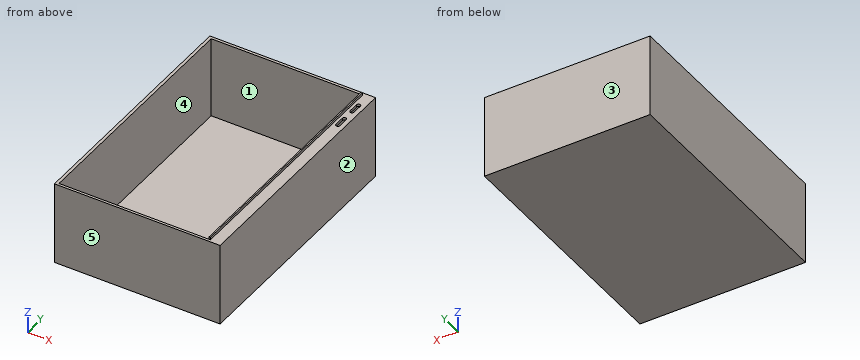
```python
from build123d import *

# Parameters (mm, degrees)
F0_W     = 406.4
F0_H     = 609.6
F1_DEPTH = 203.2
F2_W     = 368.3
F2_H     = 596.9
F3_DEPTH = 199.39
F5_DEPTH = 25.4
F7_DEPTH = 25.4
F8_W     = 3.175
F8_H     = 596.9
F9_DEPTH = 6.35


with BuildPart() as f1:
    # F0 (on Top) → F1 (new body)
    with BuildSketch(Plane.XY):
        Rectangle(F0_W, F0_H)
    extrude(amount=F1_DEPTH)

    # F2 (on face) → F3 (cut)
    with BuildSketch(Plane.XY.offset(203.2)):
        with Locations((-11.712919, -0.323749)):
            Rectangle(F2_W, F2_H)
    extrude(amount=-F3_DEPTH, mode=Mode.SUBTRACT)

    # F4 (on face) → F5 (cut)
    with BuildSketch(Plane(origin=(172.437081, 0, 0), x_dir=(0, -1, 0), z_dir=(-1, 0, 0))):
        Polygon((-298.126251, 196.85), (-298.126251, 3.81), (298.773749, 3.81), (298.773749, 196.85), (-77.169992, 196.85), align=None)
    extrude(amount=-F5_DEPTH, mode=Mode.SUBTRACT)

    # F6 (on face) → F7 (cut)
    with BuildSketch(Plane.XY.offset(203.2)):
        with BuildLine():
            Line((192.28287, 237.560081), (192.282062, 262.872214))
            ThreePointArc((192.282062, 262.872214), (187.564229, 267.722228), (182.75787, 262.959929))
            Line((182.75787, 262.959929), (182.75787, 237.559929))
            ThreePointArc((182.75787, 237.559929), (187.520446, 232.797429), (192.28287, 237.560081))
        make_face()
        with BuildLine():
            Line((192.282946, 181.997568), (192.282208, 207.31357))
            ThreePointArc((192.282208, 207.31357), (187.562377, 212.159745), (182.757946, 207.397429))
            Line((182.757946, 207.397429), (182.757946, 181.997429))
            ThreePointArc((182.757946, 181.997429), (187.520515, 177.234929), (192.282946, 181.997568))
        make_face()
    extrude(amount=-F7_DEPTH, mode=Mode.SUBTRACT)

    # F8 (on face) → F9 (join)
    with BuildSketch(Plane.XY.offset(203.2)):
        with Locations((174.024581, -0.323749)):
            Rectangle(F8_W, F8_H)
    extrude(amount=F9_DEPTH)


solid = f1.part
```
Input: part model. Units: mm. Frame: model coordinates. Face numbers are marked on the shaded views. A direction names the side the tool comes from. Coordinates: 2 decimals unless noted, no trailing zeros. Write each loop counter-clockwise with the first axis right and the second up, starting at its lowest first coordinate (ties: lowest second). Pieces come first, ordered by that corner, then holes. Notation, with made-up numbers: (58.25, 71.25) - (76.25, 71.25) arc R19 cw to (76.25, 105.25) - close; hole circle Ø3 at (57.5, 84.25). An arc over 180 degrees is marked (long way). Put each result on its own line as item: value. Start each with the question number.
1) Cut plane B-B (y = -58). Return the cut outline in (x, z), plus the area to 3 significant figures.
2) Reachability of the marked faces 4 and 5 from +Z, -Z, +X, -X, +Y, -Y: full face, straight path, thin tool, end or side. Return the list, or none.
3) Contact query for flat-ended pins moving along their axis: pin 1 (2.5 mm diameter, centred on x = 173.5, z = 207, fed in from -Y); pin 2 (6 mm diameter, centred on x = 12.5, y = 166, fed in from +Z); pin 3 (2.5 mm diameter, centred on x = 173.5, z = 206, fed in from +Y). Output: stop coordinate, or through.
4) Mould query, pull axis X, two halves, no side actions, for the marked faces 1, 2 and 3. Classes: pulls with the +X half, pulls with the -X half, needs draft (parallel to the pull), parting line crosses it, or undercut.
5) Ray query, L1, parallel to X at y = 131.5, z = 45.5; L2, parallel to Y at x = 42.5, z = 167; L3, parallel to Z at x = 84.5, y = 37. Return the intervals inside material, ascending.
6) Cut plane C-C (x = -97). Return the cut outline in (y, z), plus the area to 3 significant figures.
7) Cut plane A-A (z = 32). Return the cut outline in (x, y).
Resolved:
1. outline: (-203.2, 0) - (203.2, 0) - (203.2, 203.2) - (175.61, 203.2) - (175.61, 209.55) - (172.44, 209.55) - (172.44, 196.85) - (197.84, 196.85) - (197.84, 3.81) - (-195.86, 3.81) - (-195.86, 203.2) - (-203.2, 203.2) - close
1. area: 4,260 mm2
2. face 4: +Z
2. face 5: +Z, -Z, +X, -X, -Y
3. pin 1: stops at y = -298.77
3. pin 2: stops at z = 3.81
3. pin 3: stops at y = 298.13
4. face 1: undercut
4. face 2: pulls with the +X half
4. face 3: needs draft
5. L1: x = -203.2 to -195.86, 197.84 to 203.2
5. L2: y = -304.8 to -298.77, 298.13 to 304.8
5. L3: z = 0 to 3.81
6. outline: (-304.8, 0) - (304.8, 0) - (304.8, 203.2) - (298.13, 203.2) - (298.13, 3.81) - (-298.77, 3.81) - (-298.77, 203.2) - (-304.8, 203.2) - close
6. area: 4,850 mm2
7. outline: (-203.2, -304.8) - (203.2, -304.8) - (203.2, 304.8) - (-203.2, 304.8) - close; hole (-195.86, -298.77) - (197.84, -298.77) - (197.84, 298.13) - (-195.86, 298.13) - close
